Autodesk Inventor part; units mm, degrees
ref_plane "YZ Plane" through (0, 0, 0) normal (1, 0, 0) x (0, 1, 0)
ref_plane "XZ Plane" through (0, 0, 0) normal (0, 1, 0) x (-1, 0, 0)
ref_plane "XY Plane" through (0, 0, 0) normal (0, 0, 1) x (1, 0, 0)
sketch "스케치1" plane through (0, 0, 0) normal (0, 1, 0) x (-1, 0, 0)
  line L0 (0, 0) -> (97.5, 0)
  line L1 (97.5, 0) -> (97.5, -99.2)
  line L2 (97.5, -99.2) -> (0, -99.2)
  line L3 (0, -99.2) -> (0, 0)
  line L4 (97.5, 0) -> (1, 0)
  line L5 (1, 0) -> (1, -12)
  line L6 (1, -12) -> (97.5, -12)
  line L7 (97.5, -12) -> (97.5, 0)
  point P0 (1, -6)
  point P1 (97.5, -6)
  point P2 (48.75, 0)
  dimension "d0" = 97.5
  dimension "d1" = 99.2
  dimension "d2" = 96.5
  dimension "d3" = 12
  dimension "d6" = 1
sketch "스케치1 outline for 돌출1" plane through (0, 0, 0) normal (0, 1, 0) x (-1, 0, 0)
  line L0 (0, 0) -> (0, -99.2)
  line L1 (1, 0) -> (0, 0)
  line L2 (1, -12) -> (1, 0)
  line L3 (97.5, -12) -> (1, -12)
  line L4 (97.5, -99.2) -> (97.5, -12)
  line L5 (0, -99.2) -> (97.5, -99.2)
extrude "돌출1" add sketch "스케치1 outline for 돌출1" along normal blind 36
sketch "스케치1 outline for 돌출2" plane through (0, 0, 0) normal (0, 1, 0) x (-1, 0, 0)
  line L0 (1, -12) -> (97.5, -12)
  line L1 (1, 0) -> (1, -12)
  line L2 (97.5, 0) -> (1, 0)
  line L3 (97.5, -12) -> (97.5, 0)
extrude "돌출2" add sketch "스케치1 outline for 돌출2" along normal blind 1
sketch "스케치2" plane through (0, 1, 0) normal (0, 1, 0) x (1, 0, 0)
  circle A0 centre (-5, 4) radius 1.5
  line L0 (0, 0) -> (0, 99.2)
  line L1 (-97.5, 0) -> (-1, 0)
  line L2 (-97.5, 0) -> (0, 0)
  line L3 (-97.5, 0) -> (-87.5, 0)
  line L4 (-87.5, 0) -> (-87.5, 9)
  line L5 (-87.5, 9) -> (-97.5, 9)
  line L6 (-97.5, 9) -> (-97.5, 0)
  dimension "d11" = 3
  dimension "d13" = 5
  dimension "d14" = 4
  dimension "d15" = 10
  dimension "d16" = 9
sketch "스케치2 outline for 돌출3" plane through (0, 1, 0) normal (0, 1, 0) x (1, 0, 0)
  line L0 (-97.5, 9) -> (-97.5, 0)
  line L1 (-87.5, 9) -> (-97.5, 9)
  line L2 (-87.5, 0) -> (-87.5, 9)
  line L3 (-97.5, 0) -> (-87.5, 0)
extrude "돌출3" cut sketch "스케치2 outline for 돌출3" against normal blind 1
sketch "스케치2 outline for 돌출4" plane through (0, 1, 0) normal (0, 1, 0) x (1, 0, 0)
  line L0 (-97.5, 9) -> (-97.5, 0)
  line L1 (-87.5, 9) -> (-97.5, 9)
  line L2 (-87.5, 0) -> (-87.5, 9)
  line L3 (-97.5, 0) -> (-87.5, 0)
extrude "돌출4" add sketch "스케치2 outline for 돌출4" along normal blind 4
sketch "스케치2 outline for 돌출5" plane through (0, 1, 0) normal (0, 1, 0) x (1, 0, 0)
  line L0 (-97.5, 9) -> (-97.5, 0)
  line L1 (-87.5, 9) -> (-97.5, 9)
  line L2 (-87.5, 0) -> (-87.5, 9)
  line L3 (-97.5, 0) -> (-87.5, 0)
extrude "돌출5" cut sketch "스케치2 outline for 돌출5" along normal blind 3.4
sketch "스케치3" plane through (-87.5, 5, -9) normal (0, 0, -1) x (-1, 0, 0)
  line L0 (0, 0) -> (10, 0)
  line L1 (10, 0) -> (10, -4)
  line L2 (10, -4) -> (0, -4)
  line L3 (0, -4) -> (0, 0)
  point P0 (-87.5, -5)
  point P1 (0, -0.6)
sketch "스케치3 outline for 돌출6" plane through (-87.5, 5, -9) normal (0, 0, -1) x (-1, 0, 0)
  line L0 (0, 0) -> (0, -4)
  line L1 (10, 0) -> (0, 0)
  line L2 (10, -4) -> (10, 0)
  line L3 (0, -4) -> (10, -4)
extrude "돌출6" add sketch "스케치3 outline for 돌출6" along normal blind 0.6
chamfer "모따기1" distance 2.4 distance2 4 1 edges at (-92.5, 1, -9.6) measured on face at (-29.8333, 1, -7)
chamfer "모따기2" distance 2.4 distance2 4 1 edges at (-92.5, 0, -9)
sketch "스케치4" plane through (0, 5, 0) normal (0, 1, 0) x (1, 0, 0)
  circle A0 centre (-92.5, 4) radius 1.5
  line L0 (-97.5, 0) -> (-97.5, 9.6)
  line L1 (-97.5, 0) -> (-87.5, 0)
  point P0 (0, 0)
  point P1 (-97.5, 4.8)
  dimension "d31" = 3
  dimension "d32" = 5
  dimension "d33" = 4
sketch "스케치2 outline for 돌출7" plane through (0, 1, 0) normal (0, 1, 0) x (1, 0, 0)
  circle A0 centre (-5, 4) radius 1.5
extrude "돌출7" cut sketch "스케치2 outline for 돌출7" against normal blind 3.1
sketch "스케치4 outline for 돌출8" plane through (0, 5, 0) normal (0, 1, 0) x (1, 0, 0)
  circle A0 centre (-92.5, 4) radius 1.5
extrude "돌출8" cut sketch "스케치4 outline for 돌출8" against normal blind 3.1
sketch "스케치5" plane through (0, 0, 0) normal (1, 0, 0) x (0, 0, -1)
  circle A0 centre (18.5, 17) radius 1.5
  circle A1 centre (92.2, 17) radius 1.5
  line L0 (0, 0) -> (99.2, 0)
  line L1 (99.2, 0) -> (99.2, 36)
  circle A2 centre (6.5, 29) radius 1.5
  circle A3 centre (92.5, 29) radius 1.5
  line L2 (0, 36) -> (99.2, 36)
  line L3 (0, 0) -> (0, 36)
  line L4 (92.5, 30.5) -> (99.2, 30.5)
  line L5 (99.2, 30.5) -> (99.2, 27.5)
  line L6 (99.2, 27.5) -> (92.5, 27.5)
  line L7 (92.5, 27.5) -> (92.5, 30.5)
  dimension "d44" = 3
  dimension "d38" = 3
  dimension "d39" = 3
  dimension "d40" = 17
  dimension "d41" = 73.7
  dimension "d42" = 7
  dimension "d43" = 3
  dimension "d45" = 7
  dimension "d46" = 6.5
  dimension "d48" = 86
sketch "스케치5 outline for 돌출9" plane through (0, 0, 0) normal (1, 0, 0) x (0, 0, -1)
  circle A0 centre (6.5, 29) radius 1.5
  circle A1 centre (18.5, 17) radius 1.5
  line L0 (92.5, 27.5) -> (99.2, 27.5)
  arc A2 (92.5, 30.5) -> (92.5, 27.5) centre (92.5, 29) ccw
  line L1 (99.2, 30.5) -> (92.5, 30.5)
  line L2 (99.2, 27.5) -> (99.2, 30.5)
  circle A3 centre (92.2, 17) radius 1.5
extrude "돌출9" cut sketch "스케치5 outline for 돌출9" against normal blind 3
properties part number "smps"
For this review, take the finished solid that the model builds, in its own axes (mm). A direction names the side the tool comes from. Coordinates: 2 decimals unless noted, no trailing zeros. Order: outer loops, then holes, each group sorted by start corner. A loop starts at its lowest first (then second) coordinate and runs counter-clockwise, first axis right, second up. Notation, with made-up numbers: (79.25, -4) - (127.25, -4) arc R15 cw to (127.25, 14) - close; hole circle Ø6 at (-30.5, 3.5). An arc over 180 degrees is marked (long way). Use one line per item in the form item = value.
Q1. Draft analysis for pull direction X (two halves, no side actions). For faces 6 (the flat face through (-87.5, 4.6, -7.3)), 7 (the flat face through (-3, 17, -18)), 8 (the cylindrical face through (-6.11, 0.51, -5.01)), 9 (the cylindrical face through (-1, 17, -17)), state which applies: +X half, -X half, draft (parallel to the pull), parting line (faces both ways), or undercut.
Checked values:
face_6 = undercut
face_7 = +X half
face_8 = undercut
face_9 = draft
Q2. Consider section C-C (y = 17). Give the boundary of the cut face in (x, z), then the cut area to 3 significant figures.
Checked values:
outline = (-97.5, -99.2) - (0, -99.2) - (0, -93.7) - (-3, -93.7) - (-3, -90.7) - (0, -90.7) - (0, -20) - (-3, -20) - (-3, -17) - (0, -17) - (0, 0) - (-1, 0) - (-1, -12) - (-97.5, -12) - close
area = 8,500 mm2
Q3. For probe 1 along Y at (x, z) = (-0.2, -6.5); probe 2 along X at (y, z) = (0.75, -4); probe 3 along Y at (x, z) = (-36.5, -5.5), list the stretches that pass through material, from the lowest coordinate up. Write a range as from..to.
Checked values:
probe_1 = 0..27.5, 30.5..36
probe_2 = -87.5..-6.5, -3.5..0
probe_3 = 0..1
Q4. For P1, Ø17.5, axis at x = -51.5, y = 24.5, coming from the +Z side; P2, Ø7.5, axis at x = -93.5, z = -5, coming from the +Y side; P3, Ø3.5, axis at y = 16, z = -5.5, coming from the -X side, all flat-tipped, find the tip position at first contact; note any pin that passes through.
Checked values:
P1 = -12
P2 = 5
P3 = -1
Q5. Consider section D-D (x = -23). Give the boundary of the cut face in (y, z), then the cut area to 3 significant figures.
Checked values:
outline = (0, -99.2) - (36, -99.2) - (36, -12) - (1, -12) - (1, 0) - (0, 0) - close
area = 3,150 mm2
Q6. For faces 1 (the flat face through (0, 18, -49)), 2 (the flat face through (-3, 17, -92)), 3 (the flat face through (-93, 4.4, -6)), 4 (the flat face through (-3, 29, -95)), 5 (the flat face through (-48, 18, -99.2)), list the 3-axis set-ups (+Z, -Z, +X, -X, +Y, -Y) from which the entire face can be reached by the end or side of a thin tool; tool diameter is ignored.
Checked values:
face_1 = +Z, -Z, +X, +Y, -Y
face_2 = +X
face_3 = +Z, -X, -Y
face_4 = -Z, +X
face_5 = -Z, +X, -X, +Y, -Y
Q7. Consider section A-A (y = 29). Give the boundary of the cut face in (x, z).
Checked values:
outline = (-97.5, -99.2) - (-3, -99.2) - (-3, -91) - (0, -91) - (0, -8) - (-1, -8) - (-1, -12) - (-97.5, -12) - close; (-1, -5) - (0, -5) - (0, 0) - (-1, 0) - close
